Verification items for this drawing (mm, ordinates from the low corner). Coordinates: 2 decimals unless noted, no trailing zeros. Loops run counter-clockwise (first coordinate to the right, second up) from the corner with the lowest first, then second, coordinate; pieces in that order, holes last. Notation, with made-up numbers: (13, 48) - (65, 48) arc R21 cw to (65, 80) - close; hole circle Ø2 at (60.5, 81.25). An arc over 180 degrees is marked (long way). One line per item, written item: value. Start each with the question number.
(1) Draft check along X on the marked faces 1 and 2. Enter one of: +X half, -X half, draft (parallel to the pull), parting line (faces both ways), or undercut.
(2) Section check C-C (x = 82). Record the boundary of the cut face in (y, z), plus the area to 3 significant figures.
(3) Thickness scan on probe 1 along Y at (x, z) = (93, 2.75); probe 2 along X at (y, z) = (86.5, 3.65); probe 3 along Y at (x, z) = (16.5, 5.75). Record the ranges inside material, lowest first. Write a range as [from, to].
(4) Section check B-B (y = 86.5). Record the boundary of the cut face in (x, z), plus the area to 3 significant figures.
(5) Gauge pin test, flat ends, axial feed: P1, Ø2.5, axis at y = 58, z = 4.5, coming from the -X side; P2, Ø1, axis at x = 93.5, y = 87, coming from the +Z side; P3, Ø2.5, axis at x = 5, y = 21, coming from the +Z side. Record the tip position at first contact, or that the pin passes through.
(6) Section check A-A (z = 4). Record the boundary of the cut face in (x, y), plus the area to 3 significant figures.
(7) Section check D-D (y = 14.5). Record the boundary of the cut face in (x, z).
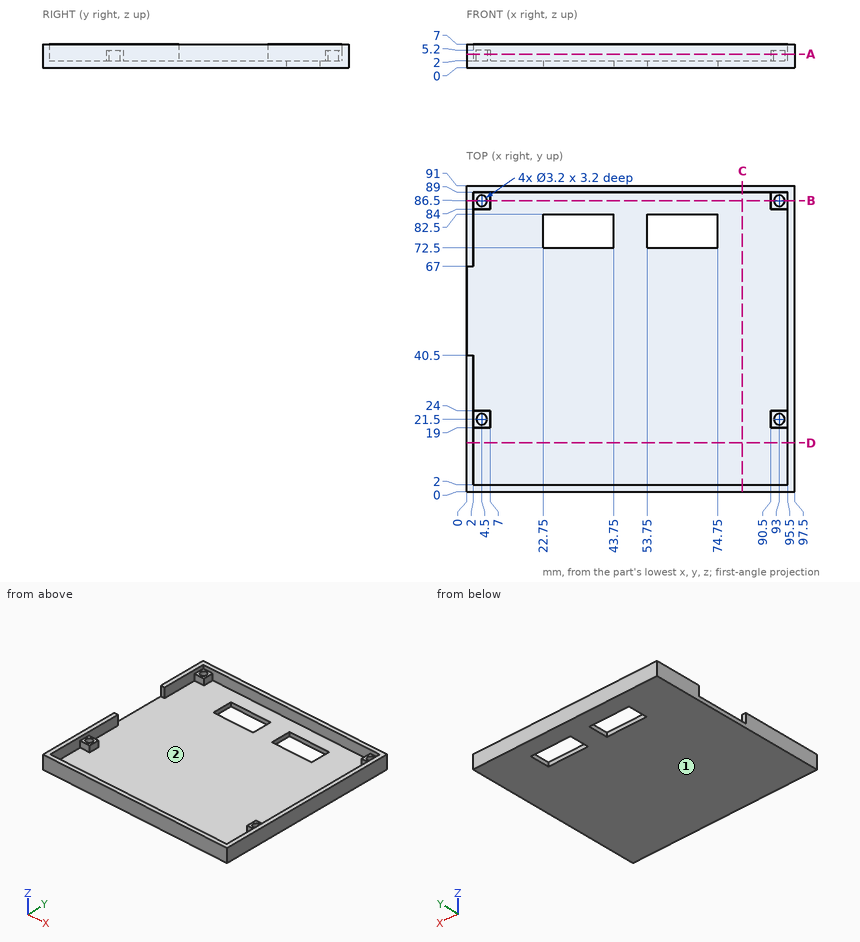
Responses:
1. face 1: draft
1. face 2: undercut
2. outline: (0, 0) - (91, 0) - (91, 7) - (89, 7) - (89, 2) - (2, 2) - (2, 7) - (0, 7) - close
2. area: 202 mm²
3. probe 1: y = [0, 2], [19, 19.9], [23.1, 24], [84, 84.9], [88.1, 91]
3. probe 2: x = [0, 2.9], [6.1, 7], [90.5, 91.4], [94.6, 97.5]
3. probe 3: y = [0, 2], [89, 91]
4. outline: (0, 0) - (97.5, 0) - (97.5, 7) - (95.5, 7) - (95.5, 5.2) - (94.6, 5.2) - (94.6, 2) - (91.4, 2) - (91.4, 5.2) - (90.5, 5.2) - (90.5, 2) - (7, 2) - (7, 5.2) - (6.1, 5.2) - (6.1, 2) - (2.9, 2) - (2.9, 5.2) - (2, 5.2) - (2, 7) - (0, 7) - close
4. area: 227 mm²
5. P1: stops at x = 95.5
5. P2: stops at z = 2
5. P3: stops at z = 5.2
6. outline: (0, 0) - (97.5, 0) - (97.5, 91) - (0, 91) - (0, 67) - (2, 67) - (2, 84) - (7, 84) - (7, 89) - (90.5, 89) - (90.5, 84) - (95.5, 84) - (95.5, 24) - (90.5, 24) - (90.5, 19) - (95.5, 19) - (95.5, 2) - (2, 2) - (2, 19) - (7, 19) - (7, 24) - (2, 24) - (2, 40.5) - (0, 40.5) - close; hole circle Ø3.2 at (4.5, 21.5); hole circle Ø3.2 at (4.5, 86.5); hole circle Ø3.2 at (93, 21.5); hole circle Ø3.2 at (93, 86.5)
6. area: 753 mm²
7. outline: (0, 0) - (97.5, 0) - (97.5, 7) - (95.5, 7) - (95.5, 2) - (2, 2) - (2, 7) - (0, 7) - close
